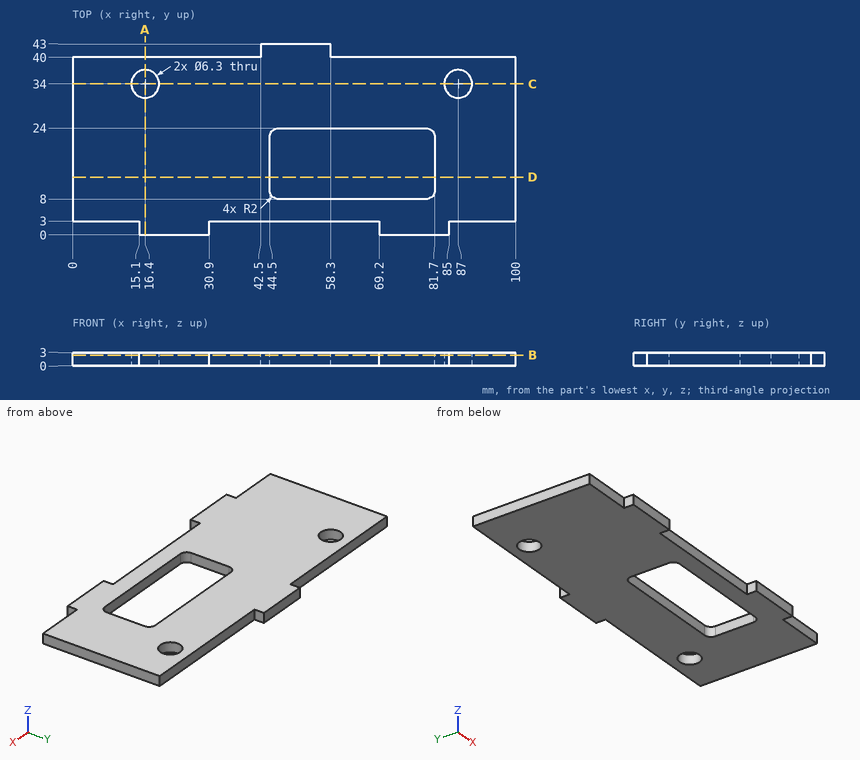
Print and shaded views of the part. All mm, measured from the part's lowest x, y and z. Round coordinates to 2 decimals unless told otherwise and drop trailing zeros. Order: outer loops, then holes, each group sorted by start corner. A loop starts at its lowest first (then second) coordinate and runs counter-clockwise, first axis right, second up.
Q1. Slice it at A-A (x = 16.4). Write the cut outline in (y, z).
Q2. Drop flat-ended pins along their axis: pin 1 (0.9 mm diameter, centred on y = 1.5, z = 2, fed in from +X); pin 2 (1.5 mm diameter, centred on x = 5, z = 2, fed in from -Y); pin 3 (0.9 mm diameter, centred on x = 21.5, z = 1, fed in from +Y). Give the stop position or say it passes through.
Q3. Wall check: L1, parallel to X at y = 17, z = 1.8; L2, parallel to X at y = 33, z = 2.1; L3, parallel to Y at x = 87, z = 1.05. Give the ranges that are in metal, low to high.
Q4. Slice it at C-C (y = 34). Write the cut outline in (x, z).
Q5. Slice it at D-D (y = 13). Write the cut outline in (x, z).
Q6. Slice it at B-B (z = 2.45). Write the cut outline in (x, y).
Results below:
1. outline: (0, 0) - (30.85, 0) - (30.85, 3) - (0, 3) - close; (37.15, 0) - (40, 0) - (40, 3) - (37.15, 3) - close
2. pin 1: stops at x = 85
2. pin 2: stops at y = 3
2. pin 3: stops at y = 40
3. L1: x = 0 to 44.5, 81.7 to 100
3. L2: x = 0 to 13.41, 19.39 to 84.01, 89.99 to 100
3. L3: y = 3 to 30.85, 37.15 to 40
4. outline: (0, 0) - (13.25, 0) - (13.25, 3) - (0, 3) - close; (19.55, 0) - (83.85, 0) - (83.85, 3) - (19.55, 3) - close; (90.15, 0) - (100, 0) - (100, 3) - (90.15, 3) - close
5. outline: (0, 0) - (44.5, 0) - (44.5, 3) - (0, 3) - close; (81.7, 0) - (100, 0) - (100, 3) - (81.7, 3) - close
6. outline: (0, 3) - (15.1, 3) - (15.1, 0) - (30.9, 0) - (30.9, 3) - (69.2, 3) - (69.2, 0) - (85, 0) - (85, 3) - (100, 3) - (100, 40) - (58.3, 40) - (58.3, 43) - (42.5, 43) - (42.5, 40) - (0, 40) - close; hole circle Ø6.3 at (16.4, 34); hole (44.5, 10) arc R2 ccw to (46.5, 8) - (79.7, 8) arc R2 ccw to (81.7, 10) - (81.7, 22) arc R2 ccw to (79.7, 24) - (46.5, 24) arc R2 ccw to (44.5, 22) - close; hole circle Ø6.3 at (87, 34)
